```python
from build123d import *

# Parameters (mm, degrees)
CROQUIS1_R              = 25
SALIENTE_EXTRUIR1_DEPTH = 2.8
CROQUIS2_W              = 2.75
CROQUIS2_H              = 18
CORTAR_EXTRUIR1_DEPTH   = 3.8
MATRIZC2_COUNT          = 5
MATRIZC2_ANGLE          = 282.12


with BuildPart() as part:
    # Croquis1 → Saliente-Extruir1 (new body)
    with BuildSketch(Plane.XY):
        Circle(CROQUIS1_R)
    extrude(amount=SALIENTE_EXTRUIR1_DEPTH)

    # Croquis2 → Cortar-Extruir1 (cut, through all)
    with BuildSketch(Plane.XY):
        with Locations((0, 25)):
            Rectangle(CROQUIS2_W, CROQUIS2_H)
    cortar_extruir1 = extrude(amount=CORTAR_EXTRUIR1_DEPTH, mode=Mode.SUBTRACT)

    # MatrizC2: Cortar-Extruir1 ×5 about axis
    matrizc2_axis = Axis((0, 0, 0), (0, 0, 1))
    for i in range(1, MATRIZC2_COUNT):
        add(cortar_extruir1.rotate(matrizc2_axis, i * MATRIZC2_ANGLE / (MATRIZC2_COUNT - 1)), mode=Mode.SUBTRACT)


solid = part.part
```
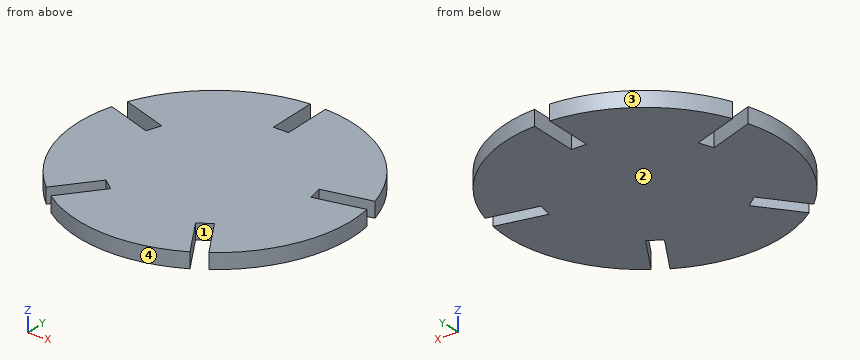
The listing builds one solid part. Answer for the finished solid, in the listing's coordinates (mm). Face numbers are marked on the shaded views. Give positions to 0.01 mm unless a question says otherwise; leave off trailing zeros. Loops run counter-clockwise (first coordinate to the right, second up) from the corner with the lowest first, then second, coordinate; pieces in that order, holes last. Notation, with made-up numbers: M 34.25,45 L 40.25,45 A9 ccw 40.25,49 Z; hole C 74,0 d5. An arc over 180 degrees is marked long. One line per item, written item: value.
1. Section B-B on y = 18.5 is taken. Determine the outline of the cut face in (x, z) (3 decimals), plus the area to 3 significant figures.
Found:
outline: M -16.815,0 L -1.375,0 L -1.375,2.8 L -16.815,2.8 Z; M 1.375,0 L 16.815,0 L 16.815,2.8 L 1.375,2.8 Z
area: 86.5 mm^2
2. Section D-D on y = -17.5 is taken. Determine the outline of the cut face in (x, z).
Found:
outline: M -17.85,0 L -15.91,0 L -15.91,2.8 L -17.85,2.8 Z; M -12.37,0 L 9.15,0 L 9.15,2.8 L -12.37,2.8 Z; M 12.38,0 L 17.85,0 L 17.85,2.8 L 12.38,2.8 Z
3. For a pull along Y with two mould halves and no side action, classify the marked faces 1, 2, 3 and 4 as pulls with the +Y half, pulls with the -Y half, needs draft (parallel to the pull), parting line crosses it, or undercut.
Found:
face 1: undercut
face 2: needs draft
face 3: pulls with the +Y half
face 4: pulls with the -Y half
4. Section A-A on x = 8 is taken. Determine the outline of the cut face in (y, z), plus the area to 3 significant figures.
Found:
outline: M -23.69,0 L -15.63,0 L -15.63,2.8 L -23.69,2.8 Z; M -13.86,0 L 23.69,0 L 23.69,2.8 L -13.86,2.8 Z
area: 128 mm^2
5. Section C-C on z = 1.9 is taken. Determine the outline of the cut face in (x, y) (1 decimal), plus the area to 3 significant figures.
Found:
outline: M -24,7 A25 ccw -16.8,-18.6 L -11.1,-11.6 L -9,-13.3 L -14.6,-20.3 A25 ccw 11.9,-22 L 7.2,-14.3 L 9.6,-12.9 L 14.2,-20.5 A25 ccw 24.7,3.9 L 15.9,2 L 15.4,4.7 L 24.1,6.6 A25 ccw 1.4,25 L 1.4,16 L -1.4,16 L -1.4,25 A25 ccw -23.1,9.6 L -14.6,6.6 L -15.5,4 Z
area: 1,840 mm^2
6. Each of these flat-tipped pins is pushed along its axis until it touches: P1, Ø0.8, axis at y = 22, z = 2, coming from the -X side; P2, Ø1, axis at x = -2.5, z = 1, coming from the -Y side; P3, Ø1.5, axis at x = 12.5, y = -19.5, coming from the -Z side; P4, Ø1, axis at y = -14, z = 2, coming from the +X side. Where does it stop, or does it pass through?
Found:
P1: x = -12.59
P2: y = -24.92
P3: through
P4: x = 21.04
7. Find the intervals of material crossed by probe 1 along X at (y, z) = (-13, 2.45); probe 2 along Y at (x, z) = (0, 1.85); probe 3 along Y at (x, z) = (11.5, 0.75), in increasing order.
Found:
probe 1: -21.35 to -12.27, -9.37 to 9.4, 9.61 to 21.35
probe 2: -25 to 16
probe 3: -22.2 to -21.33, -16.08 to 22.2
